Read the model definition and answer for the solid it produces. Units are mm, in the model's axes. A direction names the side the tool comes from. Coordinates: 2 decimals unless noted, no trailing zeros. Loops run counter-clockwise (first coordinate to the right, second up) from the corner with the lowest first, then second, coordinate; pieces in that order, holes last. Notation, with made-up numbers: (64.25, 83.5) - (90.25, 83.5) arc R7 cw to (90.25, 93.5) - close; hole circle Ø11 at (-4.75, 32.25). An arc over 180 degrees is marked (long way). Use one line per item in the form item = value.
Autodesk Inventor part; units mm, degrees
ref_plane "P1_XY" through (0, 9.5, 34.5093) normal (0, 1, 0) x (1, 0, 0)
ref_plane "P1_YZ" through (0, 9.5, 34.5093) normal (1, 0, 0) x (0, 0, -1)
ref_plane "P1_ZX" through (0, 9.5, 34.5093) normal (0, 0, -1) x (0, 1, 0)
sketch "Skizze_1" plane through (0, 0, 0) normal (0, 1, 0) x (-1, 0, 0)
  line L0 (4.7, 27.5428) -> (4.7, 40.3427)
  arc A0 (4.7, 40.3427) -> (0.7437, 44.8097) centre (0.2, 40.3427) ccw
  line L1 (0.7437, 44.8097) -> (0.5, 42.8246)
  arc A1 (2.7, 40.3427) -> (0.5, 42.8246) centre (0.2, 40.3427) ccw
  line L2 (2.7, 40.3427) -> (2.7, 27.5428)
  arc A2 (2.2372, 26.0938) -> (2.7, 27.5428) centre (0.2, 27.5428) ccw
  line L3 (2.2372, 26.0938) -> (0.4628, 23.599)
  arc A3 (0.4628, 23.599) -> (0, 22.15) centre (2.5, 22.15) ccw
  arc A4 (0, 22.15) -> (-0.4628, 23.599) centre (-2.5, 22.15) ccw
  line L4 (-0.4628, 23.599) -> (-2.2372, 26.0938)
  arc A5 (-2.7, 27.5428) -> (-2.2372, 26.0938) centre (-0.2, 27.5428) ccw
  line L5 (-2.7, 27.5428) -> (-2.7, 40.3427)
  arc A6 (-0.5, 42.8246) -> (-2.7, 40.3427) centre (-0.2, 40.3427) ccw
  line L6 (-0.5, 42.8246) -> (-0.7437, 44.8097)
  arc A7 (-0.7437, 44.8097) -> (-4.7, 40.3427) centre (-0.2, 40.3427) ccw
  line L7 (-4.7, 40.3427) -> (-4.7, 27.5428)
  arc A8 (-4.7, 27.5428) -> (-3.867, 24.9345) centre (-0.2, 27.5428) ccw
  line L8 (-3.867, 24.9345) -> (-2.0926, 22.4398)
  arc A9 (-2, 22.15) -> (-2.0926, 22.4398) centre (-2.5, 22.15) ccw
  line L9 (-2, 22.15) -> (-2, -4)
  line L10 (-2, -4) -> (2, -4)
  line L11 (2, -4) -> (2, 22.15)
  arc A10 (2.0926, 22.4398) -> (2, 22.15) centre (2.5, 22.15) ccw
  line L12 (2.0926, 22.4398) -> (3.867, 24.9345)
  arc A11 (3.867, 24.9345) -> (4.7, 27.5428) centre (0.2, 27.5428) ccw
extrude "Extrusion1" add sketch "Skizze_1" along normal mid plane 40
sketch "Skizze_2" plane through (0, 0, 0) normal (1, 0, 0) x (0, 1, 0)
  line L0 (-60, 105) -> (-60, -73)
  line L1 (-60, -73) -> (65, -73)
  line L2 (65, -73) -> (65, 105)
  line L3 (65, 105) -> (-60, 105)
  line L4 (1.5, 44.8175) -> (1.5, 22.25)
  arc A0 (-1.25, 17.7848) -> (1.5, 22.25) centre (-3.5, 22.25) ccw
  arc A1 (-1.25, 17.7848) -> (-4, 13.3197) centre (1, 13.3197) ccw
  line L5 (-4, 13.3197) -> (-4, 0)
  arc A2 (-4, 0) -> (3.9611, 0.5567) centre (0, 0) ccw
  line L6 (3.9611, 0.5567) -> (2.4717, 11.1545)
  arc A3 (7.3248, 13.908) -> (2.4717, 11.1545) centre (5.4425, 11.572) ccw
  arc A4 (7.3248, 13.908) -> (10.9583, 19.8317) centre (9.5, 16.65) ccw
  arc A5 (9.5, 22.1044) -> (10.9583, 19.8317) centre (12, 22.1044) ccw
  line L7 (9.5, 22.1044) -> (9.5, 44.8175)
  line L8 (9.5, 44.8175) -> (1.5, 44.8175)
extrude "Extrusion2" cut sketch "Skizze_2" along normal mid plane 40
sketch "Skizze_3_ALT_Drilling_1" plane through (0, 0, 0) normal (0, 1, 0) x (-1, 0, 0)
  line L0 (-10, 0) -> (10, 0)
  line L1 (10, 0) -> (10, -1.6)
  line L2 (10, -1.6) -> (-10, -1.6)
  line L3 (-10, -1.6) -> (-10, 0)
  line L4 (-10, 0) -> (10, 0)
revolve "Revolution1" cut sketch "Skizze_3_ALT_Drilling_1" angle 360 about axis through (10, 0, 0) along (1, 0, 0)
sketch "Skizze_4_ALT_Drilling_2" plane through (0, 0, 16.65) normal (0, 0, 1) x (1, 0, 0)
  line L0 (10, 9.5) -> (-10, 9.5)
  line L1 (-10, 9.5) -> (-10, 11.1)
  line L2 (-10, 11.1) -> (10, 11.1)
  line L3 (10, 11.1) -> (10, 9.5)
  line L4 (10, 9.5) -> (-10, 9.5)
revolve "Revolution2" cut sketch "Skizze_4_ALT_Drilling_2" angle 360 about axis through (10, 9.5, 16.65) along (1, 0, 0)
ref_plane "P1_XY" through (0, 9.5, 34.5093) normal (0, 1, 0) x (1, 0, 0)
ref_plane "P1_YZ" through (0, 9.5, 34.5093) normal (1, 0, 0) x (0, 0, -1)
ref_plane "P1_ZX" through (0, 9.5, 34.5093) normal (0, 0, -1) x (0, 1, 0)
ref_plane "P2_XY" through (0, 1.5, 34.5093) normal (0, 1, 0) x (1, 0, 0)
ref_plane "P2_YZ" through (0, 1.5, 34.5093) normal (1, 0, 0) x (0, 0, -1)
ref_plane "P2_ZX" through (0, 1.5, 34.5093) normal (0, 0, -1) x (0, 1, 0)
ref_plane "SA1_XY" through (0, 0, 0) normal (1, 0, 0) x (0, 0, -1)
ref_plane "SA1_YZ" through (0, 0, 0) normal (0, 0, -1) x (0, 1, 0)
ref_plane "SA1_ZX" through (0, 0, 0) normal (0, 1, 0) x (1, 0, 0)
ref_plane "SA2_XY" through (0, 9.5, 16.65) normal (1, 0, 0) x (0, 0, -1)
ref_plane "SA2_YZ" through (0, 9.5, 16.65) normal (0, 0, -1) x (0, 1, 0)
ref_plane "SA2_ZX" through (0, 9.5, 16.65) normal (0, 1, 0) x (1, 0, 0)
ref_plane "SA3_XY" through (0, 5.5, 34.5093) normal (0, 0, 1) x (1, 0, 0)
ref_plane "SA3_YZ" through (0, 5.5, 34.5093) normal (1, 0, 0) x (0, 1, 0)
ref_plane "SA3_ZX" through (0, 5.5, 34.5093) normal (0, 1, 0) x (0, 0, 1)
properties part number "305106_7-KOMP"
Item 1: The part is cut by section C-C on y = 0. Give the vertices of the cut face in (x, z), plus the area to 3 significant figures.
Results below:
outline = (-2, -4) - (2, -4) - (2, -1.6) - (-2, -1.6) - close; (-2, 1.6) - (2, 1.6) - (2, 18.68) - (-2, 18.68) - close
area = 77.9 mm²
Item 2: Each of these flat-tipped pins is pushed along its axis until it touches: P1, Ø4, axis at x = -1.5, y = -1.5, coming from the -Z side; P2, Ø2, axis at x = 2, z = 11.5, coming from the +Y side; P3, Ø5, axis at y = 0, z = 0, coming from the +X side; P4, Ø2.5, axis at x = 3, z = 37.5, coming from the -Y side. Where does it stop, or does it pass through?
Results below:
P1 = -4
P2 = 2.59
P3 = 2
P4 = 1.5
Item 3: The part is cut by section B-B on z = 37.5. Give the vertices of the cut face in (x, y).
Results below:
outline = (-4.7, 1.5) - (-2.7, 1.5) - (-2.7, 9.5) - (-4.7, 9.5) - close; (2.7, 1.5) - (4.7, 1.5) - (4.7, 9.5) - (2.7, 9.5) - close
Item 4: The part is cut by section D-D on y = 5.5. Give the vertices of the cut face in (x, z).
Results below:
outline = (-4.7, 27.54) arc R4.5 ccw to (-3.87, 24.93) - (-2.09, 22.44) arc R0.5 cw to (-2, 22.15) - (-2, 14.57) - (2, 14.57) - (2, 22.15) arc R0.5 cw to (2.09, 22.44) - (3.87, 24.93) arc R4.5 ccw to (4.7, 27.54) - (4.7, 40.34) arc R4.5 ccw to (0.74, 44.81) - (0.5, 42.82) arc R2.5 cw to (2.7, 40.34) - (2.7, 27.54) arc R2.5 cw to (2.24, 26.09) - (0.46, 23.6) arc R2.5 ccw to (0, 22.15) arc R2.5 ccw to (-0.46, 23.6) - (-2.24, 26.09) arc R2.5 cw to (-2.7, 27.54) - (-2.7, 40.34) arc R2.5 cw to (-0.5, 42.82) - (-0.74, 44.81) arc R4.5 ccw to (-4.7, 40.34) - close
Item 5: Find the intervals of material crossed by L1, parallel to X at y = 3.75, z = 34; L2, parallel to Y at x = -1.15, z = 0; L3, parallel to Y at x = 1.75, z = 17, in increasing order.
Results below:
L1 = -4.7 to -2.7, 2.7 to 4.7
L2 = -4 to -1.6, 1.6 to 4
L3 = -2.38 to 7.94, 11.06 to 12.98
Item 6: For a pull along Y with two mould halves and no side action, classify faces 6 (the cylindrical face through (2.578, 5.444, 26.772)), 7 (the flat face through (-3, 9.5, 33)), 8 (the cylindrical face through (0.03, -0.97, 1.27)) as +Y half, -Y half, draft (parallel to the pull), parting line (faces both ways), or undercut.
Results below:
face_6 = draft
face_7 = +Y half
face_8 = undercut
Item 7: The part is cut by section A-A on x = 1.25. Give the vertices of the cut face in (y, z), plus the area to 3 significant figures.
Results below:
outline = (-4, 0) arc R4 ccw (long way) to (3.96, 0.56) - (2.47, 11.15) arc R3 cw to (7.32, 13.91) arc R3.5 ccw (long way) to (10.96, 19.83) arc R2.5 cw to (9.5, 22.1) - (9.5, 24.71) - (1.5, 24.71) - (1.5, 22.25) arc R5 cw to (-1.25, 17.78) arc R5 ccw to (-4, 13.32) - close; (1.5, 42.61) - (9.5, 42.61) - (9.5, 44.72) - (1.5, 44.72) - close; hole circle Ø3.2 at (0, 0); hole circle Ø3.2 at (9.5, 16.65)
area = 252 mm²
Item 8: Which of the six approach directions +Z, -Z, +X, -X, +Y, -Y give full straight-line access (tool end or side, diameter ignored) to faces 1 (the flat face through (-3, 1.5, 34)), 2 (the flat face through (-0.624, 5.444, 43.831)), 3 (the flat face through (-2.7, 5, 34)), 4 (the flat face through (-0.028, 3.227, 5.781)), 5 (the cylindrical face through (-0.028, 3.919, 14.156))?
Results below:
face_1 = +Z, +X, -X, -Y
face_2 = +Z, +Y, -Y
face_3 = +Y, -Y
face_4 = +X, -X, +Y
face_5 = +X, -X
